CAD build for the part. Positions are in the model's coordinates, mm. A direction names the side the tool comes from. Give positions to 0.01 mm unless a question says otherwise; leave off trailing zeros. Order: outer loops, then holes, each group sorted by start corner. A loop starts at its lowest first (then second) coordinate and runs counter-clockwise, first axis right, second up.
from build123d import *

# Parameters (mm, degrees)
SZKIC2_R                    = 80
DODANIE_WYCI_GNI_CIE1_DEPTH = 52
SZKIC3_R                    = 75
WYTNIJ_WYCI_GNI_CIE1_DEPTH  = 40
SZKIC4_R                    = 70
SZKIC4_R_2                  = 65.25
DODANIE_WYCI_GNI_CIE3_DEPTH = 20
ZAOKR_GLENIE4_R             = 2
ZAOKR_GLENIE5_R             = 2
SZKIC5_W                    = 20
SZKIC5_H                    = 20
WYTNIJ_WYCI_GNI_CIE3_DEPTH  = 125.51505933


with BuildPart() as part:
    # Szkic2 → Dodanie-wyciągnięcie1 (new body)
    with BuildSketch(Plane(origin=(0, 0, 0), x_dir=(1, 0, 0), z_dir=(0, 1, 0))):
        with Locations(Location((0, 0, 0), (0, 0, 90))):
            Circle(SZKIC2_R)
    extrude(amount=DODANIE_WYCI_GNI_CIE1_DEPTH)

    # Szkic3 → Wytnij-wyciągnięcie1 (cut)
    with BuildSketch(Plane(origin=(0, 52, 0), x_dir=(1, 0, 0), z_dir=(0, 1, 0))):
        with Locations(Location((0, 0, 0), (0, 0, 270))):
            Circle(SZKIC3_R)
    extrude(amount=-WYTNIJ_WYCI_GNI_CIE1_DEPTH, mode=Mode.SUBTRACT)

    # Szkic4 → Dodanie-wyciągnięcie3 (add)
    with BuildSketch(Plane(origin=(0, 12, 0), x_dir=(1, 0, 0), z_dir=(0, 1, 0))):
        with Locations(Location((0, 0, 0), (0, 0, 270))):
            Circle(SZKIC4_R)
        with Locations(Location((0, 0, 0), (0, 0, 270))):
            Circle(SZKIC4_R_2, mode=Mode.SUBTRACT)
    extrude(amount=DODANIE_WYCI_GNI_CIE3_DEPTH)

    # Zaokrąglenie4
    zaokr_glenie4_edges = [part.edges().sort_by_distance(p)[0] for p in [
        (0, 12, -65.25),
    ]]
    fillet(zaokr_glenie4_edges, radius=ZAOKR_GLENIE4_R)

    # Zaokrąglenie5
    zaokr_glenie5_edges = [part.edges().sort_by_distance(p)[0] for p in [
        (0, 12, -70),
        (0, 12, -75),
    ]]
    fillet(zaokr_glenie5_edges, radius=ZAOKR_GLENIE5_R)

    # Szkic5 → Wytnij-wyciągnięcie3 (cut, through all)
    with BuildSketch(Plane.XZ):
        Polygon((72.116968793, -29.879745962), (89.437476869, -39.879745962), (79.437476869, -57.200254038), (62.116968793, -47.200254038), align=None)
        with Locations((0, 87.71)):
            Rectangle(SZKIC5_W, SZKIC5_H)
        Polygon((-62.116968793, -47.200254038), (-79.437476869, -57.200254038), (-89.437476869, -39.879745962), (-72.116968793, -29.879745962), align=None)
    extrude(amount=-WYTNIJ_WYCI_GNI_CIE3_DEPTH, mode=Mode.SUBTRACT)


solid = part.part
1. Saw through at B-B on y = 7. Give the cut face in (x, z).
2. 3-axis set-ups, long thin cutter, end or side, ignore diameter. For faces 5 (the cylindrical face through (-42.594, 22.874, -55.55)), 6 (the flat face through (-1, 0, 1)), 7 (the flat face through (0, 26, 77.71)): which of +Z, -Z, +X, -X, +Y, -Y reach the whole face in a straight line?
3. Saw through at C-C on x = 0. Give the cut face in (y, z), plus the area to 3 significant figures.
4. Saw through at D-D on z = 0. Give the cut face in (x, y), plus the area to 3 significant figures.
5. Wall check: line 1 (X direction, y = 28.5, z = 0); line 2 (Z direction, x = -41.5, y = 31); line 3 (X direction, y = 37.5, z = 1.5) (3 decimals). Give the ranges that are in metal, low to high.
6. Pin check, flat tips, straight feed: P1, Ø1, axis at x = -46.5, z = -40, coming from the +Y side; P2, Ø3, axis at x = -59.5, y = 31, coming from the +Z side; P3, Ø10, axis at y = 11.5, z = -57, coming from the -X side. Stop position of each tip, or through.
7. Mould opens along X. For faces 1 (the cylindrical face through (-69.75, 25.64, 39.18)), 2 (the flat face through (-48, 12, 54)), 3 (the flat face through (-54, 52, 53)), 4 (the flat face through (31.4, 32, -57.4)) say: released by +X, released by -X, zero draft, split by the parting line, or undercut.
8. Saw through at A-A on y = 39. Give the cut face in (x, z), plus the area to 3 significant figures.
Reported:
1. outline: (-73.81, -30.86) - (-72.12, -29.88) - (-62.12, -47.2) - (-63.85, -48.2) arc R80 ccw to (63.85, -48.2) - (62.12, -47.2) - (72.12, -29.88) - (73.81, -30.86) arc R80 ccw to (10, 79.37) - (10, 77.71) - (-10, 77.71) - (-10, 79.37) arc R80 ccw to start
2. face 5: +Y
2. face 6: +Z, -Z, +X, -X, -Y
2. face 7: +Z, +Y, -Y
3. outline: (0, -80) - (52, -80) - (52, -75) - (14, -75) arc R2 cw to (12, -73) - (12, -72) arc R2 cw to (14, -70) - (32, -70) - (32, -65.25) - (14, -65.25) arc R2 cw to (12, -63.25) - (12, 63.25) arc R2 cw to (14, 65.25) - (32, 65.25) - (32, 70) - (14, 70) arc R2 cw to (12, 72) - (12, 73) arc R2 cw to (14, 75) - (52, 75) - (52, 77.71) - (0, 77.71) - close
3. area: 2,400 mm2
4. outline: (-80, 0) - (80, 0) - (80, 52) - (75, 52) - (75, 14) arc R2 cw to (73, 12) - (72, 12) arc R2 cw to (70, 14) - (70, 32) - (65.25, 32) - (65.25, 14) arc R2 cw to (63.25, 12) - (-63.25, 12) arc R2 cw to (-65.25, 14) - (-65.25, 32) - (-70, 32) - (-70, 14) arc R2 cw to (-72, 12) - (-73, 12) arc R2 cw to (-75, 14) - (-75, 52) - (-80, 52) - close
4. area: 2,520 mm2
5. line 1: x = -80 to -75, -70 to -65.25, 65.25 to 70, 75 to 80
5. line 2: z = -68.39 to -62.47, -56.37 to -50.35, 50.35 to 56.37, 62.47 to 68.39
5. line 3: x = -79.986 to -74.985, 74.985 to 79.986
6. P1: stops at y = 12
6. P2: stops at z = 55.1
6. P3: stops at x = -60.79
7. face 1: released by -X
7. face 2: undercut
7. face 3: zero draft
7. face 4: undercut
8. outline: (-73.81, -30.86) - (-72.12, -29.88) - (-62.12, -47.2) - (-63.85, -48.2) arc R80 ccw to (63.85, -48.2) - (62.12, -47.2) - (72.12, -29.88) - (73.81, -30.86) arc R80 ccw to (10, 79.37) - (10, 77.71) - (-10, 77.71) - (-10, 79.37) arc R80 ccw to start; hole circle Ø150 at (0, 0)
8. area: 2,300 mm2
